Could you check a few things on this model? Use its own coordinates, in mm. A direction names the side the tool comes from. Round coordinates to 2 decimals unless told otherwise and drop trailing zeros. Write each loop counter-clockwise with the first axis right and the second up, starting at its lowest first coordinate (ties: lowest second). Pieces come first, ordered by that corner, then holes. Notation, with made-up numbers: (30.25, 76) -> (67.25, 76) arc R21 cw to (67.25, 112) -> close; hole circle Ø7 at (26.5, 49). An arc over 180 degrees is marked (long way). One line per question, with ' | ' between items. Start each with the question number.
1. Imagine slicing it at C-C, the plane z = -1.5. List the corners of the cut face in (x, y) for me.
2. Imagine slicing it at A-A, the plane y = 18. List the corners of the cut face in (x, z) for me.
3. For pin 1 Ø4.5 at (x, y) = (62, -4.5) entering from -Z; pin 2 Ø20 at (x, z) = (40.5, 44) entering from -Y; pin 3 Ø2 at (y, z) = (-7.5, 18.5) entering from -X; pin 4 Ø3 at (x, y) = (98, -26.5) entering from -Z (1 decimal), each with a flat end and sliding along its axis, tell me the tip position at first contact or that it passes through.
4. For faces 4 (the flat face through (-1, 50, 0)), 5 (the flat face through (92, 0, 38)), 6 (the cylindrical face through (44.28, -0.18, 42.49)), 7 (the flat face through (13, -5, 39)), 8 (the flat face through (63, 9, 57)), which set-ups out of +Z, -Z, +X, -X, +Y, -Y let a thin tool reach every point of the face, with its end or its side?
5. If I drill on line 1 along Z through (x, y) = (106, -5.5); line 2 along X through (y, z) = (20, 1); line 3 along Y through (x, z) = (-4, 45), over which ranges is the centre line in solid material (lowest first)? Write a range as [from, to].
6. Imagine slicing it at B-B, the plane x = 92. List the corners of the cut face in (y, z) for me, and give its area (3 significant figures).
7. Thinking about a two-plate mould opening in Z: for faces 1 (the flat face through (-1, -1, -10)), 2 (the cylindrical face through (37.518, 8.698, 49.871)), 3 (the flat face through (13, 5, 39)), which applies, released by +Z, released by -Z, zero draft, split by the parting line, or undercut?
from build123d import *

# Parameters (mm, degrees)
F1_DEPTH = 50
F2_DEPTH = 12.5
F3_DEPTH = 5
F5_DEPTH = 5


with BuildPart() as f1:
    # F0 (on Front) → F1 (new body, symmetric)
    with BuildSketch(Plane.XZ):
        Polygon((-40, -10), (40, -10), (40, 10), (30, 10), (-40, 10), align=None)
    extrude(amount=F1_DEPTH, both=True)

    # F0 (on Front) → F2 (join, symmetric)
    with BuildSketch(Plane.XZ):
        with BuildLine():
            Line((30, 10), (40, 10))
            Line((40, 10), (40, 32))
            ThreePointArc((40, 32), (44.3933982822, 42.6066017178), (55, 47))
            Line((55, 47), (67, 47))
            Line((67, 47), (67, 57))
            Line((67, 57), (55, 57))
            ThreePointArc((55, 57), (37.3223304703, 49.6776695297), (30, 32))
            Line((30, 32), (30, 10))
        make_face()
    extrude(amount=F2_DEPTH, both=True)

    # F0 (on Front) → F3 (join, symmetric)
    with BuildSketch(Plane.XZ):
        with BuildLine():
            add(Edge.make_bspline(
                [(-40, 10), (-31.567607969, 40.394651228), (11, 68.0161871854), (67, 68)],
                knots=[0, 0, 0, 0, 121.7086685491, 121.7086685491, 121.7086685491, 121.7086685491], degree=3))
            Line((-40, 10), (30, 10))
            Line((30, 10), (30, 32))
            ThreePointArc((30, 32), (37.3223304703, 49.6776695297), (55, 57))
            Line((55, 57), (67, 57))
            Line((67, 57), (67, 68))
        make_face()
    extrude(amount=F3_DEPTH, both=True)

    # F0 (on Front) → F4 (revolve)
    with BuildSketch(Plane.XZ):
        Polygon((117, 68), (92, 68), (92, 57), (92, 47), (92, 38), (117, 38), align=None)
    revolve(axis=Axis((92, 0, 52), (0, 0, -1)))

    # F5 (add): faces of the model
    f5_faces = [f1.faces().sort_by_distance(p)[0] for p in [
        (67, 5.1041666667, 55.2083333333),
        (67, -5.1041666667, 55.2083333333),
    ]]
    extrude(f5_faces, amount=F5_DEPTH)


solid = f1.part
Geometry results:
1) outline: (-40, -50) -> (40, -50) -> (40, 50) -> (-40, 50) -> close
2) outline: (-40, -10) -> (40, -10) -> (40, 10) -> (-40, 10) -> close; (74.65, 38) -> (109.35, 38) -> (109.35, 68) -> (74.65, 68) -> close
3) pin 1: stops at z = 47 | pin 2: stops at y = -12.5 | pin 3: stops at x = 30 | pin 4: passes through
4) face 4: +Z, -Z, +X, -X, +Y | face 5: -Z, +X, +Y, -Y | face 6: -Z, +Y, -Y | face 7: +Z, -X, -Y | face 8: +Z, -X, +Y
5) line 1: z = [38, 68] | line 2: x = [-40, 40] | line 3: y = [-5, 5]
6) outline: (-25, 38) -> (25, 38) -> (25, 68) -> (-25, 68) -> close | area: 1,500 mm2
7) face 1: released by -Z | face 2: released by +Z | face 3: zero draft
